Geometry: see drawing. Coordinates: mm, zero at the bounding-box minimum. A direction names the side the tool comes from. Round coordinates to 2 decimals unless told otherwise and drop trailing zeros. Write each loop counter-clockwise with the first axis right and the second up, starting at its lowest first coordinate (ties: lowest second). Pieces come first, ordered by that corner, then holes. Notation, with made-up numbers: (-25.75, -18) -> (25.25, -18) arc R19 ccw to (25.25, -1) -> close; hole circle Ø8 at (-12, 6). An arc over 180 degrees is marked (long way). Use CSV: the item, a comma, the result in double quotes.
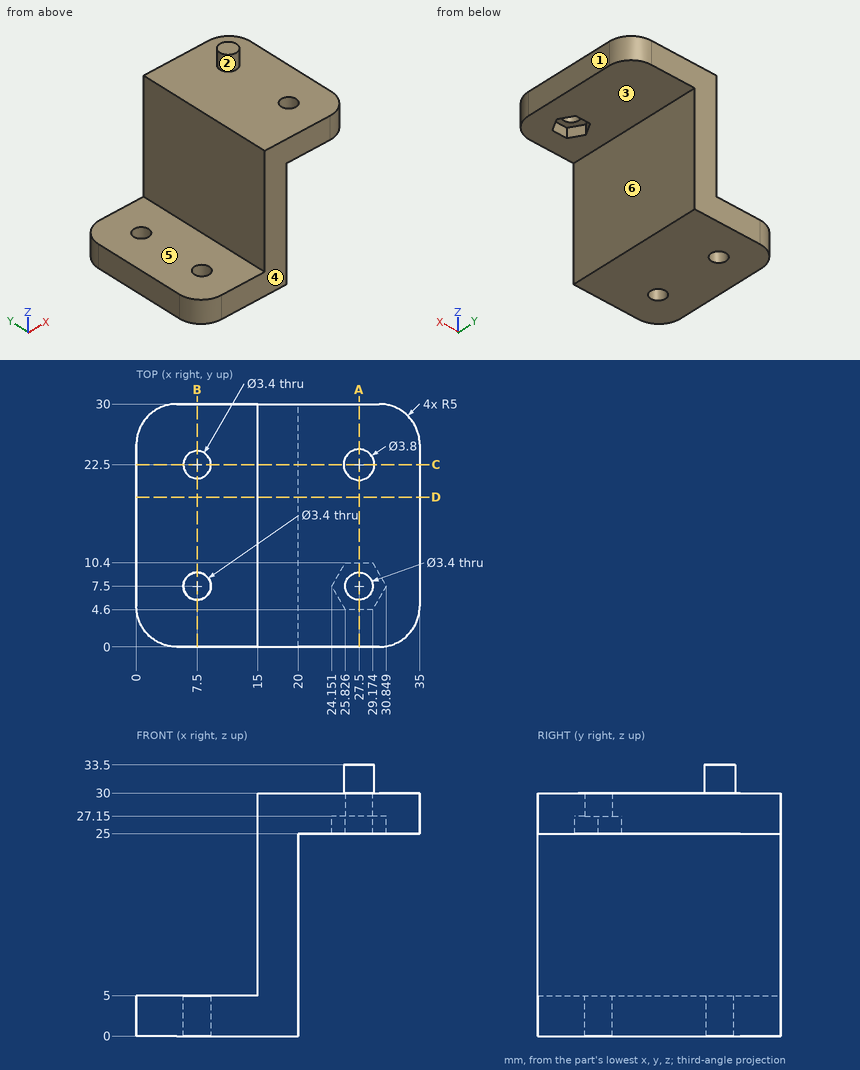
Item 1: Section query B-B on x = 7.5. Return the cut outline in (y, z).
Worked answers:
outline,"(0, 0) -> (5.8, 0) -> (5.8, 5) -> (0, 5) -> close; (9.2, 0) -> (20.8, 0) -> (20.8, 5) -> (9.2, 5) -> close; (24.2, 0) -> (30, 0) -> (30, 5) -> (24.2, 5) -> close"
Item 2: Section query C-C on y = 22.5. Return the cut outline in (x, z), plus the area to 3 significant figures.
Worked answers:
outline,"(0, 0) -> (5.8, 0) -> (5.8, 5) -> (0, 5) -> close; (9.2, 0) -> (20, 0) -> (20, 25) -> (35, 25) -> (35, 30) -> (29.4, 30) -> (29.4, 33.5) -> (25.6, 33.5) -> (25.6, 30) -> (15, 30) -> (15, 5) -> (9.2, 5) -> close"
area,"296 mm²"
Item 3: First-contact query: pin 1 Ø12 at (x, y) = (11, 15.5) entering from +Z; pin 2 Ø12 at (x, y) = (30, 11) entering from -Z; pin 3 Ø1.7 at (x, y) = (28.5, 7.5) entering from -Z. Flat tips, straight axial feed; report the tip coordinate or a pass-through.
Worked answers:
pin 1,"stops at z = 30"
pin 2,"stops at z = 25"
pin 3,"stops at z = 27.15"
Item 4: Section query D-D on y = 18.5. Return the cut outline in (x, z), plus the area to 3 significant figures.
Worked answers:
outline,"(0, 0) -> (20, 0) -> (20, 25) -> (35, 25) -> (35, 30) -> (15, 30) -> (15, 5) -> (0, 5) -> close"
area,"300 mm²"
Item 5: Pull-direction query (X, two-part tool) for the marked faces 1, 2 and 3; classes: +X half, -X half, draft (parallel to the pull), parting line (faces both ways), or undercut.
Worked answers:
face 1,"+X half"
face 2,"parting line"
face 3,"draft"
Item 6: Set-up query: the marked faces 4, 5 and 6. Return all of +Z, -Z, +X, -X, +Y, -Y with unobstructed straight access to the full face (end or side cutting, diameter ignored); none if empty.
Worked answers:
face 4,"+Z, -Z, +X, -X, -Y"
face 5,"+Z, -X, +Y, -Y"
face 6,"-Z, +X, +Y, -Y"
Item 7: Section query A-A on x = 27.5. Return the cut outline in (y, z).
Worked answers:
outline,"(0, 25) -> (4.6, 25) -> (4.6, 27.15) -> (5.8, 27.15) -> (5.8, 30) -> (0, 30) -> close; (9.2, 27.15) -> (10.4, 27.15) -> (10.4, 25) -> (30, 25) -> (30, 30) -> (24.4, 30) -> (24.4, 33.5) -> (20.6, 33.5) -> (20.6, 30) -> (9.2, 30) -> close"
Item 8: Line query: line 1 (Y direction, x = 7.5, z = 3.4); line 2 (Y direction, x = 27.5, z = 29.2); line 3 (Z direction, x = 10, y = 21). Output: solid intervals per line, ascending.
Worked answers:
line 1,"y = 0 to 5.8, 9.2 to 20.8, 24.2 to 30"
line 2,"y = 0 to 5.8, 9.2 to 30"
line 3,"z = 0 to 5"
